Here's how the part is built. I have some questions about the finished solid (model axes, mm). A direction names the side the tool comes from. Coordinates: 2 decimals unless noted, no trailing zeros. Write each loop counter-clockwise with the first axis right and the second up, starting at its lowest first coordinate (ties: lowest second). Pieces come first, ordered by that corner, then holes.
(1) Please list where these lines run through material, in increasing order: probe 1 along Y at (x, z) = (1.5, -44.45); probe 2 along X at (y, z) = (43, -69.5) (3 decimals); probe 3 along Z at (x, y) = (63.5, 46) (3 decimals).
(2) Which directions (+Z, -Z, +X, -X, +Y, -Y) give clear straight access to the entire face, cutting with the end or side of a thin tool? Please do faces 1 (the flat face through (52, 25, -3.175)), 2 (the cylindrical face through (2, 36, -43)).
(3) Imagine slicing it at C-C, the plane z = -44.45. List the corners of the cut face in (x, y) for me (3 decimals), plus the area to 3 significant figures.
(4) Imagine slicing it at D-D, the plane x = 68. List the corners of the cut face in (y, z) for me (3 decimals), plus the area to 3 significant figures.
(5) Thinking about a two-plate mould opening in X: for faces 3 (the flat face through (3.175, 25, -40)), 4 (the cylindrical face through (64.649, 11.147, -1.565)), 5 (the cylindrical face through (66.12, 35.61, -1.57)), 6 (the flat face through (28, 0, -2)), which applies, released by +X, released by -X, zero draft, split by the parting line, or undercut?
(6) Imagine slicing it at B-B, the plane z = -69.85. List the corners of the cut face in (x, y) for me (3 decimals).
(7) Imagine slicing it at A-A, the plane y = 38.1. List the corners of the cut face in (x, z) for me (3 decimals).
(8) For pin 1 Ø6 at (y, z) = (25.4, -69.85) entering from +X (3 decimals); pin 2 Ø4.5 at (x, y) = (92.075, 25.4) entering from -Z; pin 3 Ø6 at (x, y) = (53, 15) entering from -Z (3 decimals), each with a flat end and sliding along its axis, tell me the tip position at first contact or that it passes through.
```python
from build123d import *

# Parameters (mm, degrees)
BOSS_EXTRUDE1_DEPTH = 50.8
SKETCH2_R           = 2.5527
CUT_EXTRUDE1_DEPTH  = 50.8
SKETCH3_R           = 2.5527
CUT_EXTRUDE2_DEPTH  = 50.8


with BuildPart() as part:
    # Sketch1 → Boss-Extrude1 (new body)
    with BuildSketch(Plane(origin=(0, 0, 0), x_dir=(1, 0, 0), z_dir=(0, 1, 0))):
        Polygon((0, 0), (0, 76.2), (3.175, 76.2), (3.175, 3.175), (101.6, 3.175), (101.6, 0), align=None)
    extrude(amount=BOSS_EXTRUDE1_DEPTH)

    # Sketch2 → Cut-Extrude1 (cut)
    with BuildSketch(Plane.XY):
        with Locations((92.075, 25.4)):
            Circle(SKETCH2_R)
        with Locations((66.675, 38.1)):
            Circle(SKETCH2_R)
        with Locations((66.675, 12.7)):
            Circle(SKETCH2_R)
    extrude(amount=-CUT_EXTRUDE1_DEPTH, mode=Mode.SUBTRACT)

    # Sketch3 → Cut-Extrude2 (cut)
    with BuildSketch(Plane.ZY):
        with Locations((-69.85, 25.4)):
            Circle(SKETCH3_R)
        with Locations((-44.45, 38.1)):
            Circle(SKETCH3_R)
        with Locations((-44.45, 12.7)):
            Circle(SKETCH3_R)
    extrude(amount=-CUT_EXTRUDE2_DEPTH, mode=Mode.SUBTRACT)


solid = part.part
```
Recorded:
1. probe 1: y = 0 to 10.15, 15.25 to 35.55, 40.65 to 50.8
1. probe 2: x = 0 to 3.175
1. probe 3: z = -3.175 to 0
2. face 1: -Z, +X, +Y, -Y
2. face 2: +X, -X
3. outline: (0, 0) - (3.175, 0) - (3.175, 10.147) - (0, 10.147) - close; (0, 15.253) - (3.175, 15.253) - (3.175, 35.547) - (0, 35.547) - close; (0, 40.653) - (3.175, 40.653) - (3.175, 50.8) - (0, 50.8) - close
3. area: 129 mm2
4. outline: (0, -3.175) - (10.518, -3.175) - (10.518, 0) - (0, 0) - close; (14.882, -3.175) - (35.918, -3.175) - (35.918, 0) - (14.882, 0) - close; (40.282, -3.175) - (50.8, -3.175) - (50.8, 0) - (40.282, 0) - close
4. area: 134 mm2
5. face 3: released by +X
5. face 4: undercut
5. face 5: undercut
5. face 6: zero draft
6. outline: (0, 0) - (3.175, 0) - (3.175, 22.847) - (0, 22.847) - close; (0, 27.953) - (3.175, 27.953) - (3.175, 50.8) - (0, 50.8) - close
7. outline: (0, -76.2) - (3.175, -76.2) - (3.175, -47.003) - (0, -47.003) - close; (0, -41.897) - (3.175, -41.897) - (3.175, -3.175) - (64.122, -3.175) - (64.122, 0) - (0, 0) - close; (69.228, -3.175) - (101.6, -3.175) - (101.6, 0) - (69.228, 0) - close
8. pin 1: stops at x = 3.175
8. pin 2: passes through
8. pin 3: stops at z = -3.175
